Geometry check sheet. Reference: the model listing, model coordinates, mm. A direction names the side the tool comes from. Give positions to 0.01 mm unless a question says otherwise; leave off trailing zeros. Loops run counter-clockwise (first coordinate to the right, second up) from the corner with the lowest first, then second, coordinate; pieces in that order, holes last. Notation, with made-up numbers: (44.25, -11.75) -> (80.25, -11.75) arc R24 cw to (80.25, 24.25) -> close; hole circle Ø7 at (5, 5). An arc over 180 degrees is marked (long way). One line per item, written item: value. Start each with the question number.
(1) Sectioned sample at C-C, the plane x = 0. Record the cut outline in (y, z).
(2) Gauge pin test, flat ends, axial feed: pin 1 Ø8.5 at (x, z) = (0, 0) entering from +Y; pin 2 Ø4.5 at (x, z) = (2, -1) entering from -Y; pin 3 Ø3 at (x, z) = (-10, 12.5) entering from -Y. Record the tip position at first contact, or that the pin passes through.
(3) Sectioned sample at A-A, the plane x = -13.5. Record the cut outline in (y, z), then the cut area to 3 significant figures.
(4) Draft check along Y on faces 4 (the face through (-19, -2, 11)), 5 (the face through (0, -1, 10)), 6 (the face through (-10, 4, 13)), 7 (the face through (-20, 11, 0)). Enter one of: pulls with the +Y half, pulls with the -Y half, needs draft (parallel to the pull), parting line crosses it, or undercut.
(5) Sectioned sample at D-D, the plane z = 1.5. Record the cut outline in (x, y).
(6) Sectioned sample at B-B, the plane y = -3.5. Record the cut outline in (x, z).
(7) Scan lines: line 1 along Z through (x, y) = (10, -2.5); line 2 along X through (y, z) = (-2, 11.5); line 3 along Z through (x, y) = (0, -4.7). Record each from-to range of solid material in increasing order. Write a range as from..to.
(8) Tool access check on faces 1 (the face through (14, 17, 9)), 2 (the face through (-19, 1, 0)), 3 (the face through (1.5, 14, -14)). Record the directions out of +Z, -Z, +X, -X, +Y, -Y that give a thin tool (end or side, any length) a straight path to the whole face; none if there is none.
Autodesk Inventor part; units mm, degrees
ref_plane "Work Plane1" through (0, 17, 0) normal (0, 1, 0) x (-1, 0, 0)
ref_plane "YZ Plane" through (0, 0, 0) normal (1, 0, 0) x (0, 1, 0)
ref_plane "XY Plane" through (0, 0, 0) normal (0, 0, 1) x (1, 0, 0)
sketch "Sketch1" plane through (0, 0, 0) normal (0, 1, 0) x (-1, 0, 0)
  line L0 (-20, 17.5) -> (20, 17.5)
  line L1 (20, 17.5) -> (20, -17.5)
  line L2 (20, -17.5) -> (-20, -17.5)
  line L3 (-20, -17.5) -> (-20, 17.5)
  line L4 (-20, 17.5) -> (20, -17.5) construction
  line L5 (20, 17.5) -> (-20, -17.5) construction
  point P0 (0, 0)
  dimension "d0" = 35
  dimension "d1" = 40
extrude "Extrusion1" add sketch "Sketch1" along normal blind 21
sketch "Sketch2" plane through (0, 21, 0) normal (0, 1, 0) x (1, 0, 0)
  circle A0 centre (0, 0) radius 10.2
  line L0 (-1.5, 10.0891) -> (-1.5, 17.5)
  line L1 (-1.5, 17.5) -> (1.5, 17.5)
  line L2 (20, 17.5) -> (-20, 17.5)
  line L3 (1.5, 17.5) -> (1.5, 10.0891)
  line L4 (0, 0) -> (0, 17.5) construction
  dimension "d4" = 20.4
  dimension "d7" = 3
extrude "Extrusion2" cut sketch "Sketch2" against normal blind 15
sketch "Sketch3" plane through (0, 6, 0) normal (0, 1, 0) x (1, 0, 0)
  circle A0 centre (0, 0) radius 2.25
  dimension "d8" = 4.5
extrude "Extrusion3" cut sketch "Sketch3" against normal through all
sketch "Sketch5" plane through (0, 0, 0) normal (0, -1, 0) x (1, 0, 0)
  circle A0 centre (0, 0) radius 7.25
  dimension "d11" = 14.5
extrude "Extrusion4" cut sketch "Sketch5" against normal blind 3
sketch "Sketch6" plane through (0, 21, 0) normal (0, 1, 0) x (1, 0, 0)
  line L0 (-13.5, -9) -> (13.5, -9) construction
  line L1 (13.5, -9) -> (13.5, 9) construction
  line L2 (13.5, 9) -> (-13.5, 9) construction
  line L3 (-13.5, 9) -> (-13.5, -9) construction
  line L4 (-13.5, -9) -> (13.5, 9) construction
  line L5 (13.5, -9) -> (-13.5, 9) construction
  circle A0 centre (-13.5, 9) radius 5.05
  circle A1 centre (13.5, 9) radius 5.05
  circle A2 centre (13.5, -9) radius 5.05
  circle A3 centre (-13.5, -9) radius 5.05
  point P0 (0, 0)
  dimension "d14" = 18
  dimension "d15" = 27
  dimension "d16" = 10.1
ref_plane "Work Plane1" through (0, 17, 0) normal (0, 1, 0) x (-1, 0, 0)
sketch "Sketch7" plane through (0, 17, 0) normal (0, 1, 0) x (-1, 0, 0)
  circle A0 centre (13.5, -9) radius 3.65
  circle A1 centre (-13.5, -9) radius 3.65
  circle A2 centre (-13.5, 9) radius 3.65
  circle A3 centre (13.5, 9) radius 3.65
  line L0 (13.5, 9) -> (-13.5, 9) construction
  line L1 (-13.5, 9) -> (-13.5, -9) construction
  line L2 (-13.5, -9) -> (13.5, -9) construction
  line L3 (13.5, -9) -> (13.5, 9) construction
  line L4 (13.5, 9) -> (-13.5, -9) construction
  line L5 (-13.5, 9) -> (13.5, -9) construction
  point P0 (0, 0)
  dimension "d20" = 7.3
  dimension "d21" = 27
  dimension "d22" = 18
loft "Loft2" cut profiles "Sketch6", "Sketch7" contours A0 / A0
loft "Loft3" cut profiles "Sketch6", "Sketch7" contours A3 / A3
loft "Loft4" cut profiles "Sketch6", "Sketch7" contours A1 / A1
loft "Loft5" cut profiles "Sketch6", "Sketch7" contours A2 / A2
sketch "Sketch8" plane through (0, 0, 0) normal (0, -1, 0) x (1, 0, 0)
  line L0 (-20, -17.5) -> (20, -17.5)
  line L1 (20, -17.5) -> (20, -10)
  line L2 (-20, -10) -> (-20, -17.5)
  line L3 (-20, 17.5) -> (20, 17.5)
  line L4 (20, 17.5) -> (20, 10)
  line L5 (-20, 10) -> (-20, 17.5)
  line L6 (20, 10) -> (-20, 10)
  line L7 (20, -10) -> (-20, -10)
  point P0 (0, 0)
  dimension "d50" = 20
extrude "Extrusion6" add sketch "Sketch8" along normal blind 3
sketch "Sketch9" plane through (0, -3, 0) normal (0, -1, 0) x (1, 0, 0)
  line L0 (-20, 17.5) -> (20, 17.5)
  line L1 (-20, -17.5) -> (-20, 17.5)
  line L2 (20, 17.5) -> (-20, 17.5)
  line L3 (-20, 17.5) -> (-20, -17.5)
  line L4 (-20, -17.5) -> (20, -17.5)
  line L5 (20, -17.5) -> (20, 17.5)
  circle A0 centre (0, 0) radius 7.25
  arc A1 (7.25, 0) -> (7.25, 0) centre (0, 0) ccw
extrude "Extrusion7" add sketch "Sketch9" along normal blind 3
fillet "Fillet1" radius 2 4 edges at (-20, 7.5, -17.5) (-20, 7.5, 17.5) (20, 7.5, -17.5) (20, 7.5, 17.5)
chamfer "Chamfer1" distance 2 angle 45 8 edges at (-20, -3, 0) (-20, -1.5, -10) (-20, 0, 0) (-20, -1.5, 10) (20, 0, 0) (20, -1.5, 10) (20, -3, 0) (20, -1.5, -10)
sketch "Sketch10" plane through (0, -6, 0) normal (0, -1, 0) x (1, 0, 0)
  line L0 (10, 12.5) -> (-10, 12.5) construction
  line L1 (-10, 12.5) -> (-10, -12.5) construction
  line L2 (-10, -12.5) -> (10, -12.5) construction
  line L3 (10, -12.5) -> (10, 12.5) construction
  line L4 (10, 12.5) -> (-10, -12.5) construction
  line L5 (-10, 12.5) -> (10, -12.5) construction
  circle A0 centre (10, -12.5) radius 2
  circle A1 centre (10, 12.5) radius 2
  circle A2 centre (-10, 12.5) radius 2
  circle A3 centre (-10, -12.5) radius 2
  point P0 (0, 0)
  dimension "d55" = 20
  dimension "d56" = 25
  dimension "d57" = 4
extrude "Extrusion8" cut sketch "Sketch10" against normal blind 10
properties part number "Electromagnet Blocl" material "ABS Plastic"
Calculated:
1. outline: (-6, -17.5) -> (6, -17.5) -> (6, -2.25) -> (3, -2.25) -> (3, -7.25) -> (0, -7.25) -> (0, -10) -> (-3, -10) -> (-3, -7.25) -> (-6, -7.25) -> close; (-6, 7.25) -> (-3, 7.25) -> (-3, 10) -> (0, 10) -> (0, 7.25) -> (3, 7.25) -> (3, 2.25) -> (6, 2.25) -> (6, 10.2) -> (21, 10.2) -> (21, 17.5) -> (-6, 17.5) -> close
2. pin 1: stops at y = 6
2. pin 2: stops at y = 3
2. pin 3: stops at y = 4
3. outline: (-6, -17.5) -> (21, -17.5) -> (21, -14.05) -> (17, -12.65) -> (17, -5.35) -> (21, -3.95) -> (21, 3.95) -> (17, 5.35) -> (17, 12.65) -> (21, 14.05) -> (21, 17.5) -> (-6, 17.5) -> close; hole (-3, -10) -> (0, -10) -> (0, 10) -> (-3, 10) -> close
3. area: 815 mm2
4. face 4: undercut
4. face 5: undercut
4. face 6: pulls with the -Y half
4. face 7: needs draft
5. outline: (-20, -6) -> (-7.09, -6) -> (-7.09, -3) -> (-18, -3) -> (-20, -5) -> close; (-20, 2) -> (-18, 0) -> (-7.09, 0) -> (-7.09, 3) -> (-1.68, 3) -> (-1.68, 6) -> (-10.09, 6) -> (-10.09, 21) -> (-20, 21) -> close; (1.68, 3) -> (7.09, 3) -> (7.09, 0) -> (18, 0) -> (20, 2) -> (20, 21) -> (10.09, 21) -> (10.09, 6) -> (1.68, 6) -> close; (7.09, -6) -> (20, -6) -> (20, -5) -> (18, -3) -> (7.09, -3) -> close
6. outline: (-20, -15.5) arc R2 ccw to (-18, -17.5) -> (18, -17.5) arc R2 ccw to (20, -15.5) -> (20, -12) -> (18.5, -10.5) -> (18.5, 10.5) -> (20, 12) -> (20, 15.5) arc R2 ccw to (18, 17.5) -> (-18, 17.5) arc R2 ccw to (-20, 15.5) -> (-20, 12) -> (-18.5, 10.5) -> (-18.5, -10.5) -> (-20, -12) -> close; hole circle Ø4 at (-10, -12.5); hole circle Ø4 at (-10, 12.5); hole circle Ø14.5 at (0, 0); hole circle Ø4 at (10, -12.5); hole circle Ø4 at (10, 12.5)
7. line 1: z = -17.5..-14.5, -10.5..-10, 10..10.5, 14.5..17.5
7. line 2: x = -19.5..-11.73, -8.27..8.27, 11.73..19.5
7. line 3: z = -17.5..-7.25, 7.25..17.5
8. face 1: +Y
8. face 2: -X
8. face 3: -Z, +Y
